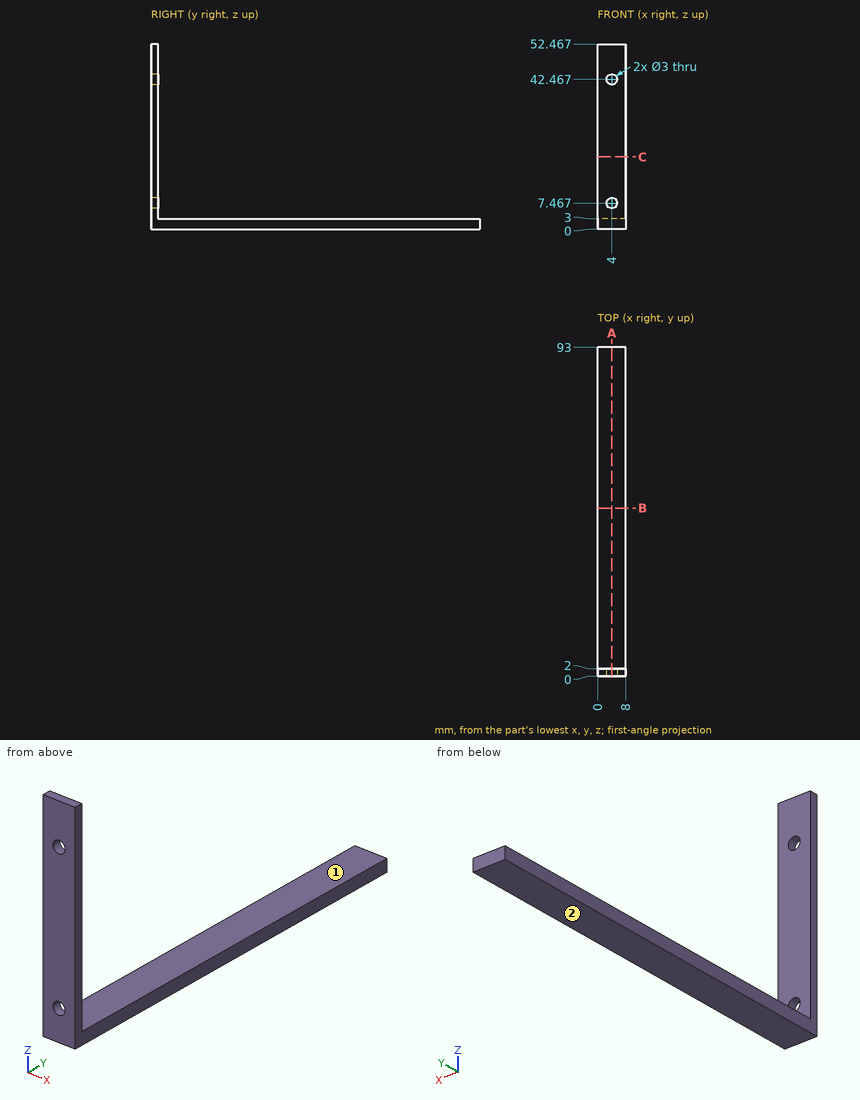
Print and shaded views of the part. All mm, measured from the part's lowest x, y and z. A direction names the side the tool comes from. Round coordinates to 2 decimals unless told otherwise and drop trailing zeros. Write each loop counter-clockwise with the first axis right and the second up, starting at its lowest first coordinate (ties: lowest second). Pieces come first, ordered by that corner, then holes. Notation, with made-up numbers: M -31,65.5 L 18,65.5 A19 ccw 18,97.5 Z; hole C 89,13.25 d11. An arc over 180 degrees is marked long. One line per question, with ' | ' between items.
(1) Saw through at C-C on z = 20.5. Write the cut outline in (x, y), then the cut area to 3 significant figures.
Answer key:
outline: M 0,0 L 8,0 L 8,2 L 0,2 Z | area: 16.0 mm^2
(2) 3-axis set-ups, long thin cutter, end or side, ignore diameter. For the marked faces 1 and 2: which of +Z, -Z, +X, -X, +Y, -Y reach the whole face in a straight line?
Answer key:
face 1: +Z, +X, -X, +Y | face 2: -Z, +X, -X, +Y, -Y
(3) Saw through at B-B on y = 47.5. Write the cut outline in (x, z), then the cut area to 3 significant figures.
Answer key:
outline: M 0,0 L 8,0 L 8,3 L 0,3 Z | area: 24.0 mm^2
(4) Saw through at A-A on x = 4. Write the cut outline in (y, z), then the cut area to 3 significant figures.
Answer key:
outline: M 0,0 L 93,0 L 93,3 L 2,3 L 2,5.97 L 0,5.97 Z; M 0,8.97 L 2,8.97 L 2,40.97 L 0,40.97 Z; M 0,43.97 L 2,43.97 L 2,52.47 L 0,52.47 Z | area: 366 mm^2
(5) Pin check, flat tips, straight feed: pin 1 (4 mm diameter, centred on x = 4.5, y = 55, fed in from +Z); pin 2 (2.5 mm diameter, centred on x = 3, z = 22, fed in from +Y). Stop position of each tip, or through.
Answer key:
pin 1: stops at z = 3 | pin 2: stops at y = 2
(6) Probe line 1 along Z through (x, y) = (4, 0.5); line 2 along Z through (x, y) = (5.25, 82.5); line 3 along Y through (x, z) = (4.5, 5.5). List the from-to ranges inside material, lowest first.
Answer key:
line 1: z = 0 to 5.97, 8.97 to 40.97, 43.97 to 52.47 | line 2: z = 0 to 3 | line 3: y = 0 to 2
